```python
from build123d import *

# Parameters (mm, degrees)
SKETCH1_W           = 200
SKETCH1_H           = 200
BOSS_EXTRUDE1_DEPTH = 10
CUT_EXTRUDE1_DEPTH  = 5
SKETCH3_W           = 61.021512422
SKETCH3_H           = 60
CUT_EXTRUDE2_DEPTH  = 142.509716981
SKETCH4_W           = 70
SKETCH4_H           = 70
CUT_EXTRUDE3_DEPTH  = 3


with BuildPart() as part:
    # Sketch1 → Boss-Extrude1 (new body)
    with BuildSketch(Plane(origin=(0, 0, 0), x_dir=(0, 0, -1), z_dir=(1, 0, 0))):
        Rectangle(SKETCH1_W, SKETCH1_H)
    extrude(amount=BOSS_EXTRUDE1_DEPTH)

    # Sketch2 → Cut-Extrude1 (cut)
    with BuildSketch(Plane.ZY):
        Polygon((36.5, -36.5), (36.5, 36.5), (25.709845909, 36.5), (5.209845909, 45.5), (-5.209845909, 45.5), (-25.709845909, 36.5), (-36.5, 36.5), (-36.5, -36.5), align=None)
    extrude(amount=-CUT_EXTRUDE1_DEPTH, mode=Mode.SUBTRACT)

    # Sketch3 → Cut-Extrude2 (cut, through all)
    with BuildSketch(Plane.ZY.offset(-5)):
        Rectangle(SKETCH3_W, SKETCH3_H)
    extrude(amount=-CUT_EXTRUDE2_DEPTH, mode=Mode.SUBTRACT)

    # Sketch4 → Cut-Extrude3 (cut)
    with BuildSketch(Plane(origin=(10, 0, 0), x_dir=(0, 0, -1), z_dir=(1, 0, 0))):
        Rectangle(SKETCH4_W, SKETCH4_H)
    extrude(amount=-CUT_EXTRUDE3_DEPTH, mode=Mode.SUBTRACT)


solid = part.part
```
Input: part model. Units: mm. Frame: model coordinates. A direction names the side the tool comes from. Round coordinates to 2 decimals unless told otherwise and drop trailing zeros. Loops run counter-clockwise (first coordinate to the right, second up) from the corner with the lowest first, then second, coordinate; pieces in that order, holes last. Notation, with made-up numbers: (-37, -29.5) - (-6, -29.5) arc R27 ccw to (-6, -11.5) - close; hole circle Ø7 at (10.25, 28). An arc over 180 degrees is marked (long way). One line per item, written item: value. Start each with the question number.
(1) Section A-A, the plane y = -13. Return loops of the section in (x, z).
(2) Access query for faces 4 (the flat face through (2, -36.5, -1)), 5 (the flat face through (0, 46, 1)), 6 (the flat face through (7, 0, 32)). Directions: +Z, -Z, +X, -X, +Y, -Y. A direction counts if a zero-diameter tool reaches every point of the face in a straight line with its end or side. Return the directions, or none.
(3) Draft query along Y for faces 1 (the flat face through (10, 46, 1)), 2 (the flat face through (5, -100, 1)), 3 (the flat face through (2, -1, 36.5)). Return one class per face: +Y half, -Y half, draft (parallel to the pull), parting line (faces both ways), or undercut.
(4) Section B-B, the plane z = 18. Return loops of the section in (x, y).
(5) Ray query, line 1 (Y direction, x = 7.75, z = -14.5); line 2 (Z direction, x = 5.5, y = -12.5). Return the intervals inside material, ascending. Write a range as [from, to].
(6) Section C-C, the plane x = 2. Return loops of the section in (y, z).
(7) Contact query for a flat-ended pin moving along its axis: P1, Ø8, axis at y = -27, z = 4.5, coming from the -X side. Output: stop coordinate, or through.
Results below:
1. outline: (0, -100) - (10, -100) - (10, -35) - (7, -35) - (7, -30.51) - (5, -30.51) - (5, -36.5) - (0, -36.5) - close; (0, 36.5) - (5, 36.5) - (5, 30.51) - (7, 30.51) - (7, 35) - (10, 35) - (10, 100) - (0, 100) - close
2. face 4: -X
2. face 5: +Z, -Z, -X, +Y, -Y
2. face 6: +X
3. face 1: draft
3. face 2: -Y half
3. face 3: undercut
4. outline: (0, -100) - (10, -100) - (10, -35) - (7, -35) - (7, -30) - (5, -30) - (5, -36.5) - (0, -36.5) - close; (0, 39.88) - (5, 39.88) - (5, 30) - (7, 30) - (7, 35) - (10, 35) - (10, 100) - (0, 100) - close
5. line 1: [-100, -35], [35, 100]
5. line 2: [-100, -30.51], [30.51, 100]
6. outline: (-100, -100) - (100, -100) - (100, 100) - (-100, 100) - close; hole (-36.5, -36.5) - (36.5, -36.5) - (36.5, -25.71) - (45.5, -5.21) - (45.5, 5.21) - (36.5, 25.71) - (36.5, 36.5) - (-36.5, 36.5) - close
7. P1: x = 5
